Verification items for the finished model (mm, model axes). A direction names the side the tool comes from. Round coordinates to 2 decimals unless told otherwise and drop trailing zeros. Order: outer loops, then holes, each group sorted by start corner. A loop starts at its lowest first (then second) coordinate and runs counter-clockwise, first axis right, second up. Notation, with made-up numbers: (-17.75, -19.5) -> (33.25, -19.5) arc R14 ccw to (33.25, -1.5) -> close; hole circle Ø2 at (74, 20). An arc over 180 degrees is marked (long way). Return JSON: item names as keys, results as strings. Group by question number.
Item 1: Sectioned sample at C-C on x = 25. Give the number of separate pieces and of enclosed holes in the cut face, plus the area to 3 significant figures.
Item 2: Draft check along Y on faces 1 (the flat face through (0, 10, 16)), 2 (the flat face through (0, 8, 0)), 3 (the flat face through (0, -10, -16)), 4 (the flat face through (0, 6, -20)). Enter one of: pulls with the +Y half, pulls with the -Y half, needs draft (parallel to the pull), parting line crosses it, or undercut.
Item 3: Sectioned sample at B-B on z = 5. Record the cut outline in (x, y).
Item 4: Scan lines: probe 1 along Z at (x, y) = (-4, -8.5); probe 2 along Y at (x, z) = (-7.5, -15); probe 3 along Y at (x, z) = (20, 13.5). Record each from-to range of solid material in increasing order. Write a range as from..to.
Item 5: Depth check by flat-ended pin: pin 1 Ø0.8 at (x, z) = (-12, 9) entering from -Y. Enter the tip coordinate at first touch or a pass-through.
Item 6: Sectioned sample at A-A on z = -1.5. Record the cut outline in (x, y), plus the area to 3 significant figures.
Item 7: Access from +Z, -Z, +X, -X, +Y, -Y to the whole of each face (thin tool, end or side, straight path). Record for faces 5 (the flat face through (0, 4, 12)), 6 (the flat face through (0, 10, -16)), 7 (the flat face through (0, -3, -19)), 8 (the flat face through (0, -8, -15)).
```python
from build123d import *

# Parameters (mm, degrees)
SKETCH11_R               = 2.1
STRUCTURAL_MEMBER1_DEPTH = 60


with BuildPart() as part:
    # Sketch11 → Structural Member1 (new body)
    with BuildSketch(Plane.YZ.offset(-30)):
        with BuildLine():
            Line((-9, -20), (-3.3, -20))
            ThreePointArc((-3.3, -20), (-3.087867966, -19.912132034), (-3, -19.7))
            Line((-3, -19.7), (-3, -18))
            Line((-3, -18), (-6, -18))
            Line((-6, -18), (-6, -17.060660172))
            Line((-6, -17.060660172), (-2.939339828, -14))
            Line((-2.939339828, -14), (-0.3, -14))
            Line((-0.3, -14), (0, -13.7))
            Line((0, -13.7), (0.3, -14))
            Line((0.3, -14), (2.939339828, -14))
            Line((2.939339828, -14), (6, -17.060660172))
            Line((6, -17.060660172), (6, -18))
            Line((6, -18), (3, -18))
            Line((3, -18), (3, -19.7))
            ThreePointArc((3, -19.7), (3.087867966, -19.912132034), (3.3, -20))
            Line((3.3, -20), (9, -20))
            ThreePointArc((9, -20), (9.707106781, -19.707106781), (10, -19))
            Line((10, -19), (10, -13.3))
            ThreePointArc((10, -13.3), (9.912132034, -13.087867966), (9.7, -13))
            Line((9.7, -13), (8, -13))
            Line((8, -13), (8, -16))
            Line((8, -16), (7.060660172, -16))
            Line((7.060660172, -16), (4, -12.939339828))
            Line((4, -12.939339828), (4, -10.3))
            Line((4, -10.3), (3.7, -10))
            Line((3.7, -10), (4, -9.7))
            Line((4, -9.7), (4, -7.060660172))
            Line((4, -7.060660172), (7.060660172, -4))
            Line((7.060660172, -4), (8, -4))
            Line((8, -4), (8, -7))
            Line((8, -7), (9.7, -7))
            ThreePointArc((9.7, -7), (9.912132034, -6.912132034), (10, -6.7))
            Line((10, -6.7), (10, 6.7))
            ThreePointArc((10, 6.7), (9.912132034, 6.912132034), (9.7, 7))
            Line((9.7, 7), (8, 7))
            Line((8, 7), (8, 4))
            Line((8, 4), (7.060660172, 4))
            Line((7.060660172, 4), (4, 7.060660172))
            Line((4, 7.060660172), (4, 9.7))
            Line((4, 9.7), (3.7, 10))
            Line((3.7, 10), (4, 10.3))
            Line((4, 10.3), (4, 12.939339828))
            Line((4, 12.939339828), (7.060660172, 16))
            Line((7.060660172, 16), (8, 16))
            Line((8, 16), (8, 13))
            Line((8, 13), (9.7, 13))
            ThreePointArc((9.7, 13), (9.912132034, 13.087867966), (10, 13.3))
            Line((10, 13.3), (10, 19))
            ThreePointArc((10, 19), (9.707106781, 19.707106781), (9, 20))
            Line((9, 20), (3.3, 20))
            ThreePointArc((3.3, 20), (3.087867966, 19.912132034), (3, 19.7))
            Line((3, 19.7), (3, 18))
            Line((3, 18), (6, 18))
            Line((6, 18), (6, 17.060660172))
            Line((6, 17.060660172), (2.939339828, 14))
            Line((2.939339828, 14), (0.3, 14))
            Line((0.3, 14), (0, 13.7))
            Line((0, 13.7), (-0.3, 14))
            Line((-0.3, 14), (-2.939339828, 14))
            Line((-2.939339828, 14), (-6, 17.060660172))
            Line((-6, 17.060660172), (-6, 18))
            Line((-6, 18), (-3, 18))
            Line((-3, 18), (-3, 19.7))
            ThreePointArc((-3, 19.7), (-3.087867966, 19.912132034), (-3.3, 20))
            Line((-3.3, 20), (-9, 20))
            ThreePointArc((-9, 20), (-9.707106781, 19.707106781), (-10, 19))
            Line((-10, 19), (-10, 13.3))
            ThreePointArc((-10, 13.3), (-9.912132034, 13.087867966), (-9.7, 13))
            Line((-9.7, 13), (-8, 13))
            Line((-8, 13), (-8, 16))
            Line((-8, 16), (-7.060660172, 16))
            Line((-7.060660172, 16), (-4, 12.939339828))
            Line((-4, 12.939339828), (-4, 10.3))
            Line((-4, 10.3), (-3.7, 10))
            Line((-3.7, 10), (-4, 9.7))
            Line((-4, 9.7), (-4, 7.060660172))
            Line((-4, 7.060660172), (-7.060660172, 4))
            Line((-7.060660172, 4), (-8, 4))
            Line((-8, 4), (-8, 7))
            Line((-8, 7), (-9.7, 7))
            ThreePointArc((-9.7, 7), (-9.912132034, 6.912132034), (-10, 6.7))
            Line((-10, 6.7), (-10, -6.7))
            ThreePointArc((-10, -6.7), (-9.912132034, -6.912132034), (-9.7, -7))
            Line((-9.7, -7), (-8, -7))
            Line((-8, -7), (-8, -4))
            Line((-8, -4), (-7.060660172, -4))
            Line((-7.060660172, -4), (-4, -7.060660172))
            Line((-4, -7.060660172), (-4, -9.7))
            Line((-4, -9.7), (-3.7, -10))
            Line((-3.7, -10), (-4, -10.3))
            Line((-4, -10.3), (-4, -12.939339828))
            Line((-4, -12.939339828), (-7.060660172, -16))
            Line((-7.060660172, -16), (-8, -16))
            Line((-8, -16), (-8, -13))
            Line((-8, -13), (-9.7, -13))
            ThreePointArc((-9.7, -13), (-9.912132034, -13.087867966), (-10, -13.3))
            Line((-10, -13.3), (-10, -19))
            ThreePointArc((-10, -19), (-9.707106781, -19.707106781), (-9, -20))
        make_face()
        with Locations((0, 10)):
            Circle(SKETCH11_R, mode=Mode.SUBTRACT)
        with Locations((0, -10)):
            Circle(SKETCH11_R, mode=Mode.SUBTRACT)
        Polygon((-8, -2.5), (-6.439339828, -2.5), (-2.939339828, -6), (2.939339828, -6), (6.439339828, -2.5), (8, -2.5), (8, 2.5), (6.439339828, 2.5), (2.939339828, 6), (-2.939339828, 6), (-6.439339828, 2.5), (-8, 2.5), align=None, mode=Mode.SUBTRACT)
    extrude(amount=STRUCTURAL_MEMBER1_DEPTH)


solid = part.part
```
Recorded:
{
 "1": {"separate pieces": "1", "enclosed holes": "3", "area": "321 mm²"},
 "2": {"face 1": "pulls with the +Y half", "face 2": "undercut", "face 3": "pulls with the -Y half", "face 4": "needs draft"},
 "3": {"outline": "(-30, -10) -> (30, -10) -> (30, -8) -> (-30, -8) -> close; (-30, -6.06) -> (30, -6.06) -> (30, -3.94) -> (-30, -3.94) -> close; (-30, 3.94) -> (30, 3.94) -> (30, 6.06) -> (-30, 6.06) -> close; (-30, 8) -> (30, 8) -> (30, 10) -> (-30, 10) -> close"},
 "4": {"probe 1": "-20..-13, -7..7, 13..20", "probe 2": "-10..-8, -6.06..-3.94, 3.94..6.06, 8..10", "probe 3": "-10..-8, -4.56..4.56, 8..10"},
 "5": {"pin 1": "y = -4"},
 "6": {"outline": "(-30, -10) -> (30, -10) -> (30, -8) -> (-30, -8) -> close; (-30, 8) -> (30, 8) -> (30, 10) -> (-30, 10) -> close", "area": "240 mm²"},
 "7": {"face 5": "+X, -X, +Y", "face 6": "+Z, -Z, +X, -X, +Y", "face 7": "-Z, +X, -X", "face 8": "+X, -X"}
}
